Drawing for the job (mm, zero at the part's lowest x, y, z). A direction names the side the tool comes from. Coordinates: 2 decimals unless noted, no trailing zeros. Write each loop counter-clockwise with the first axis right and the second up, starting at its lowest first coordinate (ties: lowest second). Pieces come first, ordered by that corner, then holes. Notation, with made-up numbers: (55.25, -37.5) -> (113.25, -37.5) arc R17 cw to (113.25, -26.5) -> close; hole circle Ø6 at (24, 61.5). An arc over 180 degrees is marked (long way). Write item = value, one per line. Start each with the question number.
Q1. Band-saw the part on B-B, the plane z = 14.25. List the corners of the cut face in (x, y) (1 decimal), plus the area to 3 significant figures.
Q2. Probe line 1 (X direction, y = 22.5, z = 20.25); line 2 (Y direction, x = 98.5, z = 6.5); line 3 (X direction, y = 34, z = 12.25) (1 decimal). List the from-to ranges inside material, lowest first.
Q3. Tool access for the marked faces 1 and 2: list every direction of +Z, -Z, +X, -X, +Y, -Y with a clear straight run to the whole face (end or side of a thin tool).
Q4. Band-saw the part on D-D, the plane x = 21.5. List the corners of the cut face in (y, z).
Q5. Band-saw the part on A-A, the plane y = 13. List the corners of the cut face in (x, z), plus the area to 3 significant figures.
Q6. Pin check, flat tips, straight feed: P1, Ø1.5, axis at x = 112, z = 11, coming from the -Y side; P2, Ø3, axis at y = 40, z = 12.5, coming from the +X side. Stop position of each tip, or through.
Q7. Band-saw the part on C-C, the plane x = 117. List the corners of the cut face in (y, z).
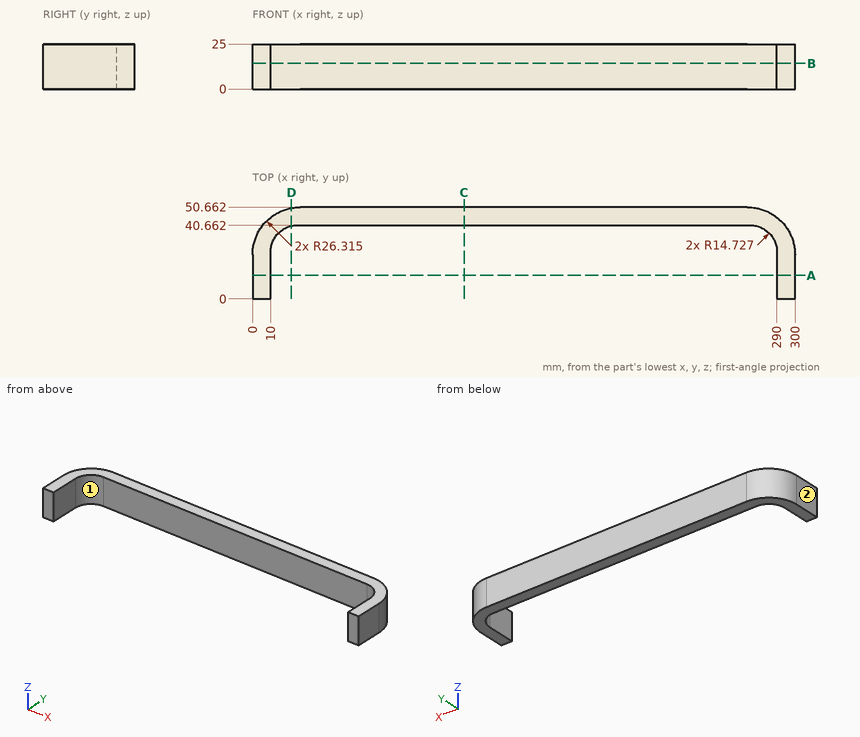
Ans:
q1.outline = (0, 0) -> (10, 0) -> (10, 25.9) arc R14.7 cw to (24.7, 40.7) -> (275.3, 40.7) arc R14.7 cw to (290, 25.9) -> (290, 0) -> (300, 0) -> (300, 24.3) arc R26.3 ccw to (273.7, 50.7) -> (26.3, 50.7) arc R26.3 ccw to (0, 24.3) -> close
q1.area = 3,610 mm2
q2.line_1 = 0 to 10, 290 to 300
q2.line_2 = 40.66 to 50.66
q2.line_3 = 1.8 to 12.4, 287.6 to 298.2
q3.face_1 = +Z, -Z, -Y
q3.face_2 = +Z, -Z, -X, +Y, -Y
q4.outline = (40.3, 0) -> (50.22, 0) -> (50.22, 25) -> (40.3, 25) -> close
q5.outline = (0, 0) -> (10, 0) -> (10, 25) -> (0, 25) -> close; (290, 0) -> (300, 0) -> (300, 25) -> (290, 25) -> close
q5.area = 500 mm2
q6.P1 = 40.66
q6.P2 = 295.87
q7.outline = (40.66, 0) -> (50.66, 0) -> (50.66, 25) -> (40.66, 25) -> close
